Design review of the part built by this model. Coordinates are the model's own, in mm. Coordinates: 2 decimals unless noted, no trailing zeros. Order: outer loops, then holes, each group sorted by start corner. A loop starts at its lowest first (then second) coordinate and runs counter-clockwise, first axis right, second up. Notation, with made-up numbers: M -37,14.25 L 6,14.25 A35 cw 6,50.25 Z; hole C 6.5,28.5 d10. An arc over 180 degrees is marked long. Answer as a JSON object with one key per item and string values.
from build123d import *

# Parameters (mm, degrees)
SZKIC1_R                    = 3.5
SZKIC1_R_2                  = 2
DODANIE_WYCI_GNI_CIE1_DEPTH = 4
SFAZOWANIE1_SIZE            = 0.2


with BuildPart() as part:
    # Szkic1 → Dodanie-wyciągnięcie1 (new body)
    with BuildSketch(Plane(origin=(0, 0, 0), x_dir=(1, 0, 0), z_dir=(0, 1, 0))):
        with Locations(Location((0, 0, 0), (0, 0, 270))):
            Circle(SZKIC1_R)
        with Locations(Location((0, 0, 0), (0, 0, 270))):
            Circle(SZKIC1_R_2, mode=Mode.SUBTRACT)
    extrude(amount=DODANIE_WYCI_GNI_CIE1_DEPTH)

    # Sfazowanie1
    sfazowanie1_edges = [part.edges().sort_by_distance(p)[0] for p in [
        (0, 0, -3.5),
        (0, 4, -3.5),
        (0, 0, -2),
        (0, 4, -2),
    ]]
    chamfer(sfazowanie1_edges, length=SFAZOWANIE1_SIZE)


solid = part.part
1) Mouldability with a two-part tool opening along Z and no side actions: class faces 1 (the cylindrical face through (-3.417, 1.975, -0.759)), 2 (the cylindrical face through (-2, 2, 0)) as released by +Z, released by -Z, zero draft, split by the parting line, or undercut.
Taken from the geometry:
{"face 1": "split by the parting line", "face 2": "undercut"}
2) Add section A-A (x = 0). State the section outline as (y, z) points.
Taken from the geometry:
{"outline": "M 0,-3.3 L 0.2,-3.5 L 3.8,-3.5 L 4,-3.3 L 4,-2.2 L 3.8,-2 L 0.2,-2 L 0,-2.2 Z; M 0,2.2 L 0.2,2 L 3.8,2 L 4,2.2 L 4,3.3 L 3.8,3.5 L 0.2,3.5 L 0,3.3 Z"}
3) Add section B-B (z = 0). State the section outline as (x, y) points, and give its area (3 significant figures).
Taken from the geometry:
{"outline": "M -3.5,0.2 L -3.3,0 L -2.2,0 L -2,0.2 L -2,3.8 L -2.2,4 L -3.3,4 L -3.5,3.8 Z; M 2,0.2 L 2.2,0 L 3.3,0 L 3.5,0.2 L 3.5,3.8 L 3.3,4 L 2.2,4 L 2,3.8 Z", "area": "11.8 mm2"}
4) Add section C-C (y = 0.4). State the section outline as (x, z) points, and give its area (3 significant figures).
Taken from the geometry:
{"outline": "C 0,0 d7; hole C 0,0 d4", "area": "25.9 mm2"}
5) To check wall thickness, follow L1, parallel to X at y = 2.55, z = 0; L2, parallel to X at y = 2.6, z = -1.75. State the ranges of each line that lie inside material, in increasing order.
Taken from the geometry:
{"L1": "x = -3.5 to -2, 2 to 3.5", "L2": "x = -3.03 to -0.97, 0.97 to 3.03"}
6) Insertion check: pin 1 Ø3 at (x, z) = (0, 0) entering from +Y; pin 2 Ø1 at (x, z) = (2, 0.5) entering from +Y. Each pin has a flat end and moves straight along its axis. Give the tip position at first contact, or say it passes through.
Taken from the geometry:
{"pin 1": "passes through", "pin 2": "stops at y = 4"}
